from build123d import *

# Parameters (mm, degrees)
F0_R        = 8
F1_DEPTH    = 2.5
F2_T1_DEPTH = 285.7168298797
F2_T3_DEPTH = 465.7168298797


# Not quite as in the source:
# - a fillet or chamfer that OpenCascade refuses, or shapes differently, is made with other operations: its cross-section is extruded or revolved along the edge and cut away or added


with BuildPart() as f1:
    # F0 (on Front) → F1 (new body)
    with BuildSketch(Plane.XZ):
        Polygon((273.1609285387, 523.1172461575), (13.1609285387, 523.1172461575), (-36.8390714613, 473.1172461575), (-36.8390714613, 33.1172461575), (13.1609285387, -16.8827538425), (273.1609285387, -16.8827538425), (323.1609285387, 33.1172461575), (323.1609285387, 473.1172461575), align=None)
        with Locations((13.1609285387, 33.1172461575)):
            Circle(F0_R, mode=Mode.SUBTRACT)
        with Locations((273.1609285387, 33.1172461575)):
            Circle(F0_R, mode=Mode.SUBTRACT)
        with Locations((13.1609285387, 473.1172461575)):
            Circle(F0_R, mode=Mode.SUBTRACT)
        with Locations((273.1609285387, 473.1172461575)):
            Circle(F0_R, mode=Mode.SUBTRACT)
    extrude(amount=F1_DEPTH)

    # F2: chamfer of 5 on 2 edges, made by hand

    # F2_s2 → F2_t1 (cut)
    with BuildSketch(Plane.YZ.offset(0.3025135989)):
        Polygon((2.5, 523.1172461575), (-2.5, 518.1172461575), (-2.5, 523.1172461575), align=None)
    extrude(amount=F2_T1_DEPTH, mode=Mode.SUBTRACT)

    # F2_s4 → F2_t3 (cut)
    with BuildSketch(Plane.XY.offset(20.2588312177)):
        Polygon((-36.8390714613, 2.5), (-31.8390714613, -2.5), (-36.8390714613, -2.5), align=None)
    extrude(amount=F2_T3_DEPTH, mode=Mode.SUBTRACT)


solid = f1.part
Geometry: final body of the model. Coordinates: model frame, mm. Round coordinates to 2 decimals unless told otherwise and drop trailing zeros. Order: outer loops, then holes, each group sorted by start corner. A loop starts at its lowest first (then second) coordinate and runs counter-clockwise, first axis right, second up. Notation, with made-up numbers: (82.5, 7) - (87.5, 7) arc R19 cw to (87.5, 27) - close; hole circle Ø9 at (41.5, 81). An arc over 180 degrees is marked (long way). Write each question's results on one line, items separated by ' | '.
Item 1: Material intervals for line 1 along Z through (x, y) = (17.5, -0.7); line 2 along X through (y, z) = (-2.3, 480); line 3 along Z through (x, y) = (67.5, -1.7), sorted ascending. Write a range as [from, to].
Completed:
line 1: [-16.88, 26.4], [39.84, 466.4], [479.84, 519.92] | line 2: [-29.96, 9.08], [17.24, 269.08], [277.24, 316.28] | line 3: [-16.88, 518.92]
Item 2: Section B-B, the plane x = -3. Return the cut outline in (y, z), and give its area (3 significant figures).
Completed:
outline: (-2.5, -0.72) - (0, -0.72) - (0, 506.96) - (-2.5, 506.96) - close | area: 1,270 mm^2
Item 3: Mould query, pull axis X, two halves, no side actions, for faces 1 (the flat face through (297.811, -1.232, 7.767)), 2 (the flat face through (-10.92, -1.23, 7.2)), 3 (the cylindrical face through (265.17, -1.23, 33.47)). Classes: pulls with the +X half, pulls with the -X half, needs draft (parallel to the pull), parting line crosses it, or undercut.
Completed:
face 1: pulls with the +X half | face 2: pulls with the -X half | face 3: undercut
Item 4: First-contact query: pin 1 Ø1.5 at (x, y) = (14.5, -1.5) entering from +Z; pin 2 Ø13 at (x, z) = (13.16, 473.12) entering from +Y. Flat tips, straight axial feed; report the tip coordinate or a pass-through.
Completed:
pin 1: z = 519.87 | pin 2: through
Item 5: Section A-A, the plane y = -0.75. Return the cut outline in (x, z).
Completed:
outline: (-33.59, 29.87) - (13.16, -16.88) - (273.16, -16.88) - (323.16, 33.12) - (323.16, 473.12) - (276.41, 519.87) - (9.91, 519.87) - (-33.59, 476.37) - close; hole circle Ø16 at (13.16, 33.12); hole circle Ø16 at (13.16, 473.12); hole circle Ø16 at (273.16, 33.12); hole circle Ø16 at (273.16, 473.12)
